```python
from build123d import *

# Parameters (mm, degrees)
F1_DEPTH = 101.6
F0_W     = 25.4
F0_H     = 25.4
F0_R     = 3.81
F2_DEPTH = 3.175


# Not quite as in the source:
# - a feature names something its author has since deleted; it is built from what else it names


with BuildPart() as f1:
    # F0 (on Front) → F1 (new body)
    with BuildSketch(Plane.XZ):
        Polygon((0, 25.4), (0, 0), (3.175, 0), (3.175, 1828.8), (917.575, 1828.8), (917.575, 0), (920.75, 0), (920.75, 25.4), (920.75, 50.8), (920.75, 318.0291666667), (920.75, 343.4291666667), (920.75, 610.6583333333), (920.75, 636.0583333333), (920.75, 903.2875), (920.75, 928.6875), (920.75, 1195.9166666667), (920.75, 1221.3166666667), (920.75, 1488.5458333333), (920.75, 1513.9458333333), (920.75, 1781.175), (920.75, 1806.575), (920.75, 1831.975), (895.35, 1831.975), (869.95, 1831.975), (613.8333333333, 1831.975), (588.4333333333, 1831.975), (332.3166666667, 1831.975), (306.9166666667, 1831.975), (50.8, 1831.975), (25.4, 1831.975), (0, 1831.975), (0, 1806.575), (0, 1781.175), (0, 1513.9458333333), (0, 1488.5458333333), (0, 1221.3166666667), (0, 1195.9166666667), (0, 928.6875), (0, 903.2875), (0, 636.0583333333), (0, 610.6583333333), (0, 343.4291666667), (0, 318.0291666667), (0, 50.8), align=None)
    extrude(amount=F1_DEPTH)

    # F0 (on Front) → F2 (join)
    with BuildSketch(Plane.XZ):
        with Locations((-12.7, 38.1)):
            Rectangle(F0_W, F0_H)
        with Locations((-12.7, 38.1)):
            Circle(F0_R, mode=Mode.SUBTRACT)
        with Locations((-12.7, 330.7291666667)):
            Rectangle(F0_W, F0_H)
        with Locations((-12.7, 330.7291666667)):
            Circle(F0_R, mode=Mode.SUBTRACT)
        with Locations((-12.7, 623.3583333333)):
            Rectangle(F0_W, F0_H)
        with Locations((-12.7, 623.3583333333)):
            Circle(F0_R, mode=Mode.SUBTRACT)
        with Locations((933.45, 38.1)):
            Rectangle(F0_W, F0_H)
        with Locations((933.45, 38.1)):
            Circle(F0_R, mode=Mode.SUBTRACT)
        with Locations((-12.7, 915.9875)):
            Rectangle(F0_W, F0_H)
        with Locations((-12.7, 915.9875)):
            Circle(F0_R, mode=Mode.SUBTRACT)
        with Locations((933.45, 330.7291666667)):
            Rectangle(F0_W, F0_H)
        with Locations((933.45, 330.7291666667)):
            Circle(F0_R, mode=Mode.SUBTRACT)
        with Locations((-12.7, 1208.6166666667)):
            Rectangle(F0_W, F0_H)
        with Locations((-12.7, 1208.6166666667)):
            Circle(F0_R, mode=Mode.SUBTRACT)
        with Locations((933.45, 623.3583333333)):
            Rectangle(F0_W, F0_H)
        with Locations((933.45, 623.3583333333)):
            Circle(F0_R, mode=Mode.SUBTRACT)
        with Locations((-12.7, 1501.2458333333)):
            Rectangle(F0_W, F0_H)
        with Locations((-12.7, 1501.2458333333)):
            Circle(F0_R, mode=Mode.SUBTRACT)
        with Locations((933.45, 915.9875)):
            Rectangle(F0_W, F0_H)
        with Locations((933.45, 915.9875)):
            Circle(F0_R, mode=Mode.SUBTRACT)
        with Locations((-12.7, 1793.875)):
            Rectangle(F0_W, F0_H)
        with Locations((-12.7, 1793.875)):
            Circle(F0_R, mode=Mode.SUBTRACT)
        with Locations((933.45, 1208.6166666667)):
            Rectangle(F0_W, F0_H)
        with Locations((933.45, 1208.6166666667)):
            Circle(F0_R, mode=Mode.SUBTRACT)
        with Locations((38.1, 1844.675)):
            Rectangle(F0_W, F0_H)
        with Locations((38.1, 1844.675)):
            Circle(F0_R, mode=Mode.SUBTRACT)
        with Locations((933.45, 1501.2458333333)):
            Rectangle(F0_W, F0_H)
        with Locations((933.45, 1501.2458333333)):
            Circle(F0_R, mode=Mode.SUBTRACT)
        with Locations((319.6166666667, 1844.675)):
            Rectangle(F0_W, F0_H)
        with Locations((319.6166666667, 1844.675)):
            Circle(F0_R, mode=Mode.SUBTRACT)
        with Locations((933.45, 1793.875)):
            Rectangle(F0_W, F0_H)
        with Locations((933.45, 1793.875)):
            Circle(F0_R, mode=Mode.SUBTRACT)
        with Locations((601.1333333333, 1844.675)):
            Rectangle(F0_W, F0_H)
        with Locations((601.1333333333, 1844.675)):
            Circle(F0_R, mode=Mode.SUBTRACT)
        with Locations((882.65, 1844.675)):
            Rectangle(F0_W, F0_H)
        with Locations((882.65, 1844.675)):
            Circle(F0_R, mode=Mode.SUBTRACT)
    extrude(amount=F2_DEPTH)


solid = f1.part
```
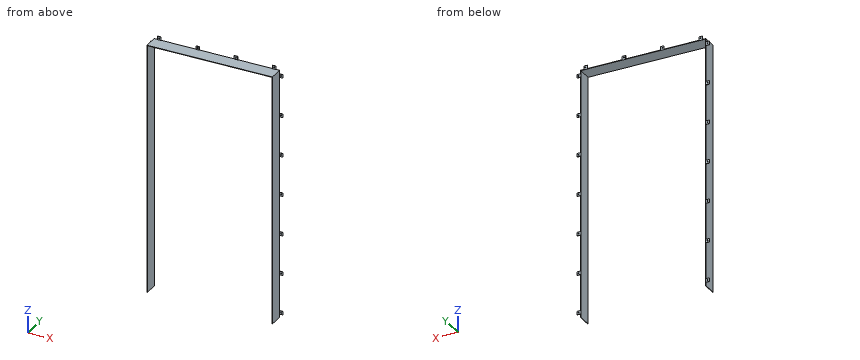
Check sheet for the modelled part. Datum: model origin and axes. Units: mm. Round coordinates to 2 decimals unless told otherwise and drop trailing zeros. Loops run counter-clockwise (first coordinate to the right, second up) from the corner with the lowest first, then second, coordinate; pieces in that order, holes last. Notation, with made-up numbers: (7, 6) -> (47, 6) arc R18 ccw to (47, 14) -> close; hole circle Ø6 at (7.5, 12.25). An arc over 180 degrees is marked (long way). Answer in a Markdown table with one row per item.
Q1. Go/stop test with flat-tipped pins: P1, Ø12, axis at x = 933.45, z = 38.1, coming from the +Y side; P2, Ø6, axis at x = -12.7, z = 1793.875, coming from the -Y side; P3, Ø2.5, axis at x = 929.5, y = -1.5, coming from the -Z side; P4, Ø12, axis at y = -84, z = 1591.5, coming from the +X side. Record where each tip stops, or that it passes through.
Data:
| item | result |
|---|---|
| P1 | stops at y = 0 |
| P2 | passes through |
| P3 | stops at z = 25.4 |
| P4 | stops at x = 920.75 |
Q2. Thickness scan on L1, parallel to Z at x = 882.65, y = -1.25 (3 decimals); L2, parallel to X at y = -39, z = 1325 (3 decimals); L3, parallel to Z at x = 269.5, y = -30 (3 decimals). Record the ranges inside material, lowest first.
Data:
| item | result |
|---|---|
| L1 | z = 1828.8 to 1840.865, 1848.485 to 1857.375 |
| L2 | x = 0 to 3.175, 917.575 to 920.75 |
| L3 | z = 1828.8 to 1831.975 |
Q3. Sectioned sample at C-C on x = 435. Enter the section's corners in (y, z) (3 decimals).
Data:
| item | result |
|---|---|
| outline | (-101.6, 1828.8) -> (0, 1828.8) -> (0, 1831.975) -> (-101.6, 1831.975) -> close |
Q4. Sectioned sample at B-B on y = -35.5. Enter the section's corners in (x, z) (3 decimals), then the cut area to 3 significant figures.
Data:
| item | result |
|---|---|
| outline | (0, 0) -> (3.175, 0) -> (3.175, 1828.8) -> (917.575, 1828.8) -> (917.575, 0) -> (920.75, 0) -> (920.75, 1831.975) -> (0, 1831.975) -> close |
| area | 14,500 mm^2 |
Q5. Sectioned sample at A-A on z = 1465. Enter the section's corners in (x, y) (3 decimals), then the cut area to 3 significant figures.
Data:
| item | result |
|---|---|
| outline | (0, -101.6) -> (3.175, -101.6) -> (3.175, 0) -> (0, 0) -> close; (917.575, -101.6) -> (920.75, -101.6) -> (920.75, 0) -> (917.575, 0) -> close |
| area | 645 mm^2 |
